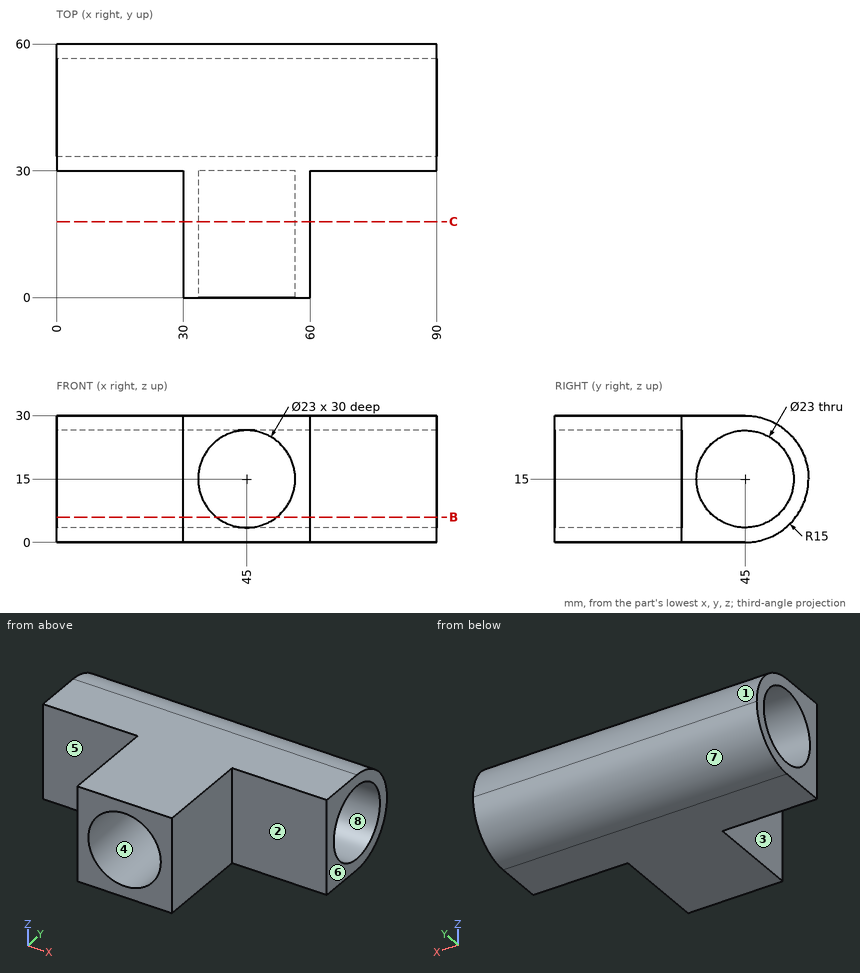
Geometry: see drawing. Coordinates: mm, zero at the bounding-box minimum. A direction names the side the tool comes from. Coordinates: 2 decimals unless noted, no trailing zeros. Loops run counter-clockwise (first coordinate to the right, second up) from the corner with the lowest first, then second, coordinate; pieces in that order, holes last.
Q1. Cut plane C-C (y = 18). Output: boundary loops of the cut face in (x, z).
Q2. Contact query for flat-ended pins moving along their axis: pin 1 (15 mm diameter, centred on y = 8, z = 10, fed in from +X); pin 2 (12 mm diameter, centred on y = 13.5, z = 8.5, fed in from -X); pin 3 (7 mm diameter, centred on x = 49.5, z = 18, fed in from -Y); pin 4 (6 mm diameter, centred on x = 34, y = 45.5, fed in from -Z). Output: stop coordinate, or through.
Q3. Material intervals for line 1 (Z direction, x = 35, y = 45); line 2 (X direction, y = 29, z = 13); line 3 (X direction, y = 13, z = 23), sorted ascending.
Q4. Cut plane B-B (z = 6). Output: boundary loops of the cut face in (x, y), then the cut area to 3 significant figures.
Q5. Draft query along Y for the marked faces 5, 6, 7 and 8. Return one class per face: +Y half, -Y half, draft (parallel to the pull), parting line (faces both ways), or undercut.
Q6. Set-up query: the marked faces 1, 2, 3 and 4. Return all of +Z, -Z, +X, -X, +Y, -Y with unobstructed straight access to the full face (end or side cutting, diameter ignored); none if empty.
Working result:
1. outline: (30, 0) - (60, 0) - (60, 30) - (30, 30) - close; hole circle Ø23 at (45, 15)
2. pin 1: stops at x = 60
2. pin 2: stops at x = 30
2. pin 3: stops at y = 30
2. pin 4: stops at z = 0
3. line 1: z = 0 to 3.5, 26.5 to 30
3. line 2: x = 30 to 33.68, 56.32 to 60
3. line 3: x = 30 to 36.74, 53.26 to 60
4. outline: (0, 30) - (30, 30) - (30, 0) - (37.84, 0) - (37.84, 30) - (52.16, 30) - (52.16, 0) - (60, 0) - (60, 30) - (90, 30) - (90, 37.84) - (0, 37.84) - close; (0, 52.16) - (90, 52.16) - (90, 57) - (0, 57) - close
4. area: 1,610 mm2
5. face 5: -Y half
5. face 6: draft
5. face 7: +Y half
5. face 8: undercut
6. face 1: +Z, +X, -X, +Y
6. face 2: +Z, -Z, +X, -Y
6. face 3: +Z, -Z, -X, -Y
6. face 4: -Y
